Can you work these out from the model? Positions are in its coordinate system, mm. A direction names the side the tool comes from. Coordinates: 2 decimals unless noted, no trailing zeros. Write each loop counter-clockwise with the first axis right and the second up, starting at its lowest first coordinate (ties: lowest second). Pieces come first, ordered by that corner, then holes. Notation, with made-up numbers: (79.5, 43.25) -> (105.5, 43.25) arc R9 cw to (105.5, 49.25) -> close; hole circle Ø11 at (12, 11). An arc over 180 degrees is marked (long way). Use one line per item in the form item = value.
Autodesk Inventor part; units mm, degrees
ref_plane "YZ Plane" through (0, 0, 0) normal (1, 0, 0) x (0, 1, 0)
ref_plane "XZ Plane" through (0, 0, 0) normal (0, 1, 0) x (-1, 0, 0)
ref_plane "XY Plane" through (0, 0, 0) normal (0, 0, 1) x (1, 0, 0)
sketch "Sketch2" plane through (0, 0, 0) normal (1, 0, 0) x (0, 1, 0)
  line L0 (0, 0) -> (59.3152, 0)
  line L1 (-40, 0) -> (40, 0)
  line L2 (40, 0) -> (40, -8.825)
  line L3 (40, -8.825) -> (-40, -8.825)
  line L4 (-40, -8.825) -> (-40, 0)
  line L5 (-1.5, -8.825) -> (1.5, -8.825)
  line L6 (1.5, -8.825) -> (1.5, -10.025)
  line L7 (1.5, -10.025) -> (-1.5, -10.025)
  line L8 (-1.5, -10.025) -> (-1.5, -8.825)
  point P0 (0, -10.025)
  point P1 (0, -8.825)
  dimension "d2" = 8.825
  dimension "d3" = 40
  dimension "d4" = 40
  dimension "d5" = 3
  dimension "d6" = 10.025
revolve "Revolution1" add sketch "Sketch2" angle 360 about axis through (0, 0, 0) along (0, 1, 0)
chamfer "Chamfer1" distance 1 distance2 3 1 edges at (0, 40, 8.825) measured on face at (2.071, 40, -2.6902)
chamfer "Chamfer2" distance 3 distance2 1 1 edges at (0, -40, 8.825) measured on face at (1.4156, -27.1667, -8.7107)
properties part number "stange_verbinder"
Q1. Will these pins go through, and if not, where does the flat tip stop? pin 1 (6 mm diameter, centred on x = -5.5, y = 22, fed in from -Z); pin 2 (2 mm diameter, centred on x = 7, y = -5.5, fed in from +Z); pin 3 (10 mm diameter, centred on y = 26, z = -5, fed in from -X) (3 decimals).
Return value:
pin_1 = -8.46
pin_2 = 6.47
pin_3 = -8.825
Q2. Suppose I cut it at A-A (z = 0). Write out the boundary of the cut face in (x, y) (3 decimals), then the cut area to 3 significant figures.
Return value:
outline = (-10.025, -1.5) -> (-8.825, -1.5) -> (-8.825, -37) -> (-7.825, -40) -> (7.825, -40) -> (8.825, -37) -> (8.825, -1.5) -> (10.025, -1.5) -> (10.025, 1.5) -> (8.825, 1.5) -> (8.825, 37) -> (7.825, 40) -> (-7.825, 40) -> (-8.825, 37) -> (-8.825, 1.5) -> (-10.025, 1.5) -> close
area = 1,410 mm2
Q3. Suppose I cut it at C-C (y = -9). Write out the boundary of the cut face in (x, z) (3 decimals), then the cut area to 3 significant figures.
Return value:
outline = circle Ø17.65 at (0, 0)
area = 245 mm2
Q4. Suppose I cut it at B-B (x = 0). Write out the boundary of the cut face in (y, z) (3 decimals).
Return value:
outline = (-40, -7.825) -> (-37, -8.825) -> (-1.5, -8.825) -> (-1.5, -10.025) -> (1.5, -10.025) -> (1.5, -8.825) -> (37, -8.825) -> (40, -7.825) -> (40, 7.825) -> (37, 8.825) -> (1.5, 8.825) -> (1.5, 10.025) -> (-1.5, 10.025) -> (-1.5, 8.825) -> (-37, 8.825) -> (-40, 7.825) -> close
Q5. For faces 1 (the cylindrical face through (-6.1, -0.021, 7.955)), 2 (the cylindrical face through (-5.37, -19.498, 7.003)), 3 (the flat face through (9, 1.5, 0)), which set-ups out of +Z, -Z, +X, -X, +Y, -Y let a thin tool reach every point of the face, with its end or its side?
Return value:
face_1 = +Y, -Y
face_2 = -Y
face_3 = +Y
Q6. If I drill on line 1 (Y direction, x = -6.5, z = -7.25); line 2 (X direction, y = 31, z = 0.5); line 3 (X direction, y = -4, z = 1.75), over which ranges is the centre line in solid material (lowest first)? Write a range as from..to.
Return value:
line_1 = -1.5..1.5
line_2 = -8.81..8.81
line_3 = -8.65..8.65
